Can you work these out from the model? Positions are in its coordinate system, mm. A direction names the side the tool comes from. Coordinates: 2 decimals unless noted, no trailing zeros. Order: outer loops, then holes, each group sorted by start corner. A loop starts at its lowest first (then second) coordinate and runs counter-clockwise, first axis right, second up. Notation, with made-up numbers: (-28, 19) -> (-13, 19) arc R21 cw to (-13, 57) -> close; hole circle Ø9 at (61.25, 74). An arc over 180 degrees is marked (long way). Answer as a JSON object with one key per item and string values. Group by question number.
(1) I want a section at C-C, the plane x = -80.5. List the corners of the cut face in (y, z) for me, plus the area to 3 significant figures.
(2) I need wall thicknesses on line 1 (X direction, y = 38, z = -46); line 2 (Z direction, x = -53.5, y = -16.5); line 3 (X direction, y = 41, z = 7). Which ranges of each line are inside material? Lowest first, please.
(3) I want a section at D-D, the plane y = 38. List the corners of the cut face in (x, z) for me, plus the area to 3 significant figures.
(4) If we mould it in two halves opening along Y, with no side actions, what happens to faces 4 (the flat face through (-69.7, -1, 9)), 5 (the flat face through (-30, -30.6, -5)), 6 (the flat face through (-47, -50.75, -20))? For each: pulls with the +Y half, pulls with the -Y half, needs draft (parallel to the pull), parting line crosses it, or undercut.
(5) Which directions (+Z, -Z, +X, -X, +Y, -Y) give clear straight access to the entire face, cutting with the end or side of a thin tool? Please do faces 1 (the flat face through (-30, -33, -24)), 2 (the cylindrical face through (-83.5, 39.6, -44.8)), 3 (the cylindrical face through (26.4, -38.16, -4.93)).
(6) For pin 1 (10 mm diameter, centred on x = -59.5, y = -4.5, fed in from -Z); pin 2 (9.5 mm diameter, centred on y = -13, z = -47, fed in from +X); pin 3 (16.5 mm diameter, centred on x = 21, y = -37.5, fed in from +Z); pin 4 (9 mm diameter, centred on x = -80.5, y = 38, fed in from -Z), each with a flat end and sliding along its axis, tell me the tip position at first contact or that it passes through.
(7) I want a section at A-A, the plane y = 0. List the corners of the cut face in (x, z) for me.
(8) I want a section at B-B, the plane z = -22.5. List the corners of the cut face in (x, y) for me.
from build123d import *

# Parameters (mm, degrees)
SKETCH_W              = 101.5
SKETCH_H              = 127
PAD_DEPTH             = 38.1
SKETCH001_W           = 101.5
SKETCH001_H           = 25.3
PAD001_DEPTH          = 19
PAD001_DEPTH_BACK     = 57
SKETCH002_R           = 3.4
POCKET_DEPTH          = 25
POCKET001_DEPTH       = 10
CLONE_ROLL_ANGLE      = 180
CLONE_PLACEMENT_ANGLE = 90


with BuildPart() as part:
    # Sketch → Pad (new body)
    with BuildSketch(Plane.XY):
        with Locations((0, -31.5)):
            Rectangle(SKETCH_W, SKETCH_H)
        with BuildLine():
            ThreePointArc((23, 1), (0, 24), (-23, 1))
            Line((-23, 1), (-23, -5))
            ThreePointArc((-23, -5), (0, -28), (23, -5))
            Line((23, 1), (23, -5))
        make_face(mode=Mode.SUBTRACT)
        with BuildLine():
            ThreePointArc((-33, 19), (-38, 24), (-43, 19))
            Line((-43, 19), (-43, 13))
            ThreePointArc((-43, 13), (-38, 8), (-33, 13))
            Line((-33, 19), (-33, 13))
        make_face(mode=Mode.SUBTRACT)
        with BuildLine():
            ThreePointArc((43, 19), (38, 24), (33, 19))
            Line((33, 19), (33, 13))
            ThreePointArc((33, 13), (38, 8), (43, 13))
            Line((43, 19), (43, 13))
        make_face(mode=Mode.SUBTRACT)
        with BuildLine():
            ThreePointArc((43, -27), (38, -22), (33, -27))
            Line((33, -27), (33, -33))
            ThreePointArc((33, -33), (38, -38), (43, -33))
            Line((43, -27), (43, -33))
        make_face(mode=Mode.SUBTRACT)
        with BuildLine():
            ThreePointArc((-33, -27), (-38, -22), (-43, -27))
            Line((-43, -27), (-43, -33))
            ThreePointArc((-43, -33), (-38, -38), (-33, -33))
            Line((-33, -27), (-33, -33))
        make_face(mode=Mode.SUBTRACT)
    extrude(amount=PAD_DEPTH)

    # Sketch001 (on Face26 of Pad) → Pad001 (join, two sides)
    with BuildSketch(Plane.XY.offset(38.1)) as pad001_sk:
        with Locations((0, -82.35)):
            Rectangle(SKETCH001_W, SKETCH001_H)
    extrude(amount=PAD001_DEPTH)
    extrude(pad001_sk.sketch, amount=-PAD001_DEPTH_BACK)

    # Sketch002 (on Face36 of Pad001) → Pocket (cut)
    with BuildSketch(Plane.XY.offset(57.1)):
        with Locations((-38, -80.5)):
            Circle(SKETCH002_R)
        with Locations((38, -80.5)):
            Circle(SKETCH002_R)
    extrude(amount=-POCKET_DEPTH, mode=Mode.SUBTRACT)

    # Sketch003 (on Face4 of Pocket) → Pocket001 (cut)
    with BuildSketch(Plane(origin=(0, 0, 0), x_dir=(1, 0, 0), z_dir=(0, 0, -1))):
        with BuildLine():
            ThreePointArc((-30.6, 33), (-38, 40.4), (-45.4, 33))
            Line((-45.4, 33), (-45.4, 27))
            ThreePointArc((-45.4, 27), (-38, 19.6), (-30.6, 27))
            Line((-30.6, 33), (-30.6, 27))
        make_face()
        with BuildLine():
            ThreePointArc((45.4, 33), (38, 40.4), (30.6, 33))
            Line((30.6, 33), (30.6, 27))
            ThreePointArc((30.6, 27), (38, 19.6), (45.4, 27))
            Line((45.4, 33), (45.4, 27))
        make_face()
        with BuildLine():
            ThreePointArc((45.4, -13), (38, -5.6), (30.6, -13))
            Line((30.6, -13), (30.6, -19))
            ThreePointArc((30.6, -19), (38, -26.4), (45.4, -19))
            Line((45.4, -13), (45.4, -19))
        make_face()
        with BuildLine():
            ThreePointArc((-30.6, -13), (-38, -5.6), (-45.4, -13))
            Line((-45.4, -13), (-45.4, -19))
            ThreePointArc((-45.4, -19), (-38, -26.4), (-30.6, -19))
            Line((-30.6, -13), (-30.6, -19))
        make_face()
    extrude(amount=-POCKET001_DEPTH, mode=Mode.SUBTRACT)


with BuildPart() as part_1:
    # Clone roll: moved
    add(part.part.rotate(Axis((0, 0, 0), (1, 0, 0)), CLONE_ROLL_ANGLE))


with BuildPart() as part_2:
    # Clone placement: moved
    add(part_1.part.rotate(Axis((0, 0, 0), (0, 0, 1)), CLONE_PLACEMENT_ANGLE))


solid = part_2.part
Computed values:
{
 "1": {"outline": "(-50.75, -57.1) -> (-41.4, -57.1) -> (-41.4, -32.1) -> (-34.6, -32.1) -> (-34.6, -57.1) -> (34.6, -57.1) -> (34.6, -32.1) -> (41.4, -32.1) -> (41.4, -57.1) -> (50.75, -57.1) -> (50.75, 18.9) -> (-50.75, 18.9) -> close", "area": "7,370 mm2"},
 "2": {"line 1": "x = -95 to -83.9, -77.1 to -69.7", "line 2": "z = -38.1 to 0", "line 3": "x = -95 to -69.7"},
 "3": {"outline": "(-95, -57.1) -> (-83.9, -57.1) -> (-83.9, -32.1) -> (-77.1, -32.1) -> (-77.1, -57.1) -> (-69.7, -57.1) -> (-69.7, -38.1) -> (-38, -38.1) -> (-38, -10) -> (-40.4, -10) -> (-40.4, 0) -> (-69.7, 0) -> (-69.7, 18.9) -> (-95, 18.9) -> close; (-22, -38.1) -> (8, -38.1) -> (8, -10) -> (5.6, -10) -> (5.6, 0) -> (-19.6, 0) -> (-19.6, -10) -> (-22, -10) -> close; (24, -38.1) -> (32, -38.1) -> (32, 0) -> (26.4, 0) -> (26.4, -10) -> (24, -10) -> close", "area": "4,310 mm2"},
 "4": {"face 4": "needs draft", "face 5": "undercut", "face 6": "pulls with the -Y half"},
 "5": {"face 1": "+Z, -Z", "face 2": "-Z", "face 3": "+Z"},
 "6": {"pin 1": "stops at z = -38.1", "pin 2": "stops at x = -69.7", "pin 3": "stops at z = 0", "pin 4": "stops at z = -57.1"},
 "7": {"outline": "(-95, -57.1) -> (-69.7, -57.1) -> (-69.7, -38.1) -> (-28, -38.1) -> (-28, 0) -> (-69.7, 0) -> (-69.7, 18.9) -> (-95, 18.9) -> close; (24, -38.1) -> (32, -38.1) -> (32, 0) -> (24, 0) -> close"},
 "8": {"outline": "(-95, -50.75) -> (32, -50.75) -> (32, 50.75) -> (-95, 50.75) -> close; hole (-33, -43) -> (-27, -43) arc R5 ccw to (-27, -33) -> (-33, -33) arc R5 ccw to start; hole (-33, 33) -> (-27, 33) arc R5 ccw to (-27, 43) -> (-33, 43) arc R5 ccw to start; hole (-5, -23) -> (1, -23) arc R23 ccw to (1, 23) -> (-5, 23) arc R23 ccw to start; hole (13, -43) -> (19, -43) arc R5 ccw to (19, -33) -> (13, -33) arc R5 ccw to start; hole (13, 33) -> (19, 33) arc R5 ccw to (19, 43) -> (13, 43) arc R5 ccw to start"}
}
